from build123d import *

# Parameters (mm, degrees)
SKETCH_1_W          = 320
SKETCH_1_H          = 150
EXTRUDE_1_DEPTH     = 40
SHELL_1_T           = -2
SKETCH_2_R          = 2.25
CUT_EXTRUDE_1_DEPTH = 2


with BuildPart() as part:
    # 草图1 → 凸台-拉伸1 (new body)
    with BuildSketch(Plane(origin=(0, 0, 0), x_dir=(1, 0, 0), z_dir=(0, 1, 0))):
        with Locations((160, 75)):
            Rectangle(SKETCH_1_W, SKETCH_1_H)
    extrude(amount=EXTRUDE_1_DEPTH)

    # 抽壳1
    shell_1_openings = [part.faces().sort_by_distance(p)[0] for p in [
        (160, 40, -75),
    ]]
    offset(amount=SHELL_1_T, openings=shell_1_openings, kind=Kind.INTERSECTION)

    # 草图2 → 切除-拉伸1 (cut)
    with BuildSketch(Plane(origin=(0, 0, 0), x_dir=(-1, 0, 0), z_dir=(0, -1, 0))):
        with Locations((-100, 55)):
            Circle(SKETCH_2_R)
        with Locations((-220, 55)):
            Circle(SKETCH_2_R)
        with Locations((-220, 120)):
            Circle(SKETCH_2_R)
        with Locations((-100, 120)):
            Circle(SKETCH_2_R)
    extrude(amount=-CUT_EXTRUDE_1_DEPTH, mode=Mode.SUBTRACT)


solid = part.part
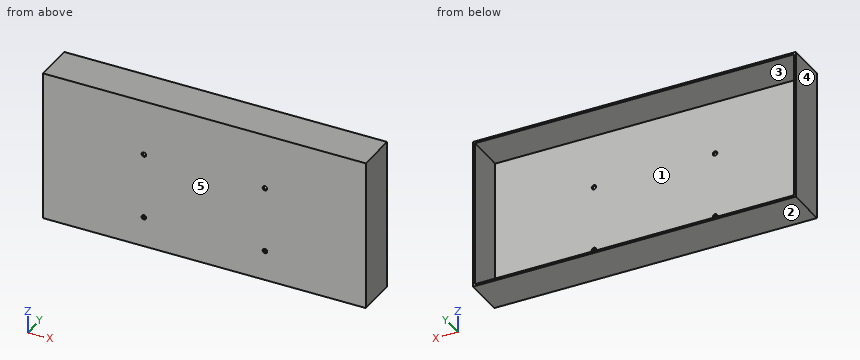
Source: CAD feature listing. Evaluate the final solid. Frame: model axes, mm. Face numbers are marked on the shaded views. A direction names the side the tool comes from. Coordinates: 2 decimals unless noted, no trailing zeros. Order: outer loops, then holes, each group sorted by start corner. A loop starts at its lowest first (then second) coordinate and runs counter-clockwise, first axis right, second up. Notation, with made-up numbers: M 55.25,-0.5 L 94.25,-0.5 A17 cw 94.25,17.5 Z; hole C 80,58 d8. An arc over 180 degrees is marked long. Write each question's results on one line, items separated by ' | '. Start each with the question number.
Item 1: Line query: probe 1 along Z at (x, y) = (220, 1.15); probe 2 along X at (y, z) = (1, -55); probe 3 along X at (y, z) = (24.5, -113). Output: solid intervals per line, ascending.
Item 2: Cut plane B-B (x = 110). Return loops of the section in (y, z), and give its area (3 significant figures).
Item 3: Cut plane C-C (z = -10). Return loops of the section in (x, y).
Item 4: Draft query along X for the marked faces 3, 4 and 5. Return one class per face: pulls with the +X half, pulls with the -X half, needs draft (parallel to the pull), parting line crosses it, or undercut.
Item 5: Set-up query: the marked faces 1 and 2. Return all of +Z, -Z, +X, -X, +Y, -Y with unobstructed straight access to the full face (end or side cutting, diameter ignored); none if empty.
Item 6: Cut plane A-A (y = 25.5). Return loops of the section in (x, z), and give its area (3 significant figures).
Item 7: First-contact query: pin 1 Ø3 at (x, z) = (127, -76) entering from +Y. Flat tip, straight axial feed; report the tip coordinate or a pass-through.
Checked values:
1) probe 1: z = -150 to -122.25, -117.75 to -57.25, -52.75 to 0 | probe 2: x = 0 to 97.75, 102.25 to 217.75, 222.25 to 320 | probe 3: x = 0 to 2, 318 to 320
2) outline: M 0,-150 L 40,-150 L 40,-148 L 2,-148 L 2,-2 L 40,-2 L 40,0 L 0,0 Z | area: 452 mm2
3) outline: M 0,0 L 320,0 L 320,40 L 318,40 L 318,2 L 2,2 L 2,40 L 0,40 Z
4) face 3: undercut | face 4: pulls with the -X half | face 5: needs draft
5) face 1: +Y | face 2: -Z, +X, -X, +Y, -Y
6) outline: M 0,-150 L 320,-150 L 320,0 L 0,0 Z; hole M 2,-148 L 318,-148 L 318,-2 L 2,-2 Z | area: 1,860 mm2
7) pin 1: stops at y = 2
